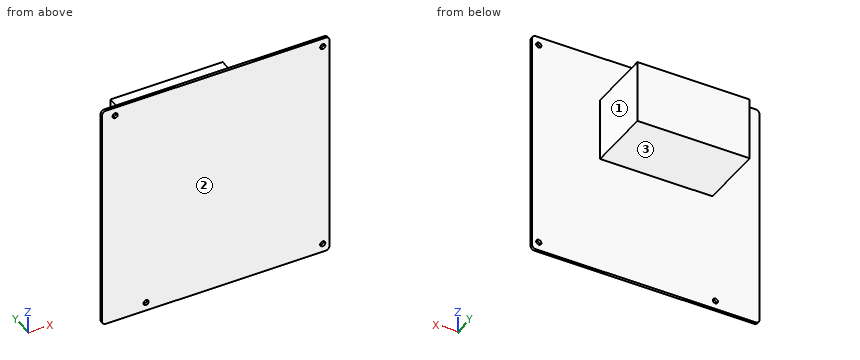
from build123d import *

# Parameters (mm, degrees)
SKETCH1_W                      = 170.18
SKETCH1_H                      = 170.18
BOSS_EXTRUDE1_DEPTH            = 2
SKETCH2_W                      = 84.015738727
SKETCH2_H                      = 47.018762818
BOSS_EXTRUDE2_DEPTH            = 48.8
FILLET1_R                      = 3
F_3_9_3_9_DIAMETER_HOLE1_D     = 3.9
F_3_9_3_9_DIAMETER_HOLE1_DEPTH = 18.75
F_3_9_3_9_DIAMETER_HOLE1_TIP   = 1.171678207


with BuildPart() as part:
    # Sketch1 → Boss-Extrude1 (new body)
    with BuildSketch(Plane(origin=(0, 0, 0), x_dir=(1, 0, 0), z_dir=(0, 1, 0))):
        Rectangle(SKETCH1_W, SKETCH1_H)
    extrude(amount=BOSS_EXTRUDE1_DEPTH)

    # Sketch2 → Boss-Extrude2 (add)
    with BuildSketch(Plane(origin=(0, 2, 0), x_dir=(1, 0, 0), z_dir=(0, 1, 0))):
        with Locations((-7.871346986, -27.578797891)):
            Rectangle(SKETCH2_W, SKETCH2_H)
    extrude(amount=BOSS_EXTRUDE2_DEPTH)

    # Fillet1
    fillet1_edges = [part.edges().sort_by_distance(p)[0] for p in [
        (-85.09, 1, -85.09),
        (85.09, 1, -85.09),
        (85.09, 1, 85.09),
        (-85.09, 1, 85.09),
    ]]
    fillet(fillet1_edges, radius=FILLET1_R)

    # Ø3.9 (3.9) Diameter Hole1
    with Locations(Plane(origin=(0, 2, 0), x_dir=(1, 0, 0), z_dir=(0, 1, 0))):
        with Locations((-75.29, -78.74), (80.01, -78.74), (80.01, 78.74), (-52.07, 78.74)):
            Hole(F_3_9_3_9_DIAMETER_HOLE1_D / 2, depth=F_3_9_3_9_DIAMETER_HOLE1_DEPTH)
            with Locations((0, 0, -(F_3_9_3_9_DIAMETER_HOLE1_DEPTH + F_3_9_3_9_DIAMETER_HOLE1_TIP / 2))):  # 118° drill point
                Cone(0, F_3_9_3_9_DIAMETER_HOLE1_D / 2, F_3_9_3_9_DIAMETER_HOLE1_TIP, mode=Mode.SUBTRACT)


solid = part.part
Geometry: final body of the model. Coordinates: model frame, mm. Face numbers are marked on the shaded views. A direction names the side the tool comes from. Round coordinates to 2 decimals unless told otherwise and drop trailing zeros. Loops run counter-clockwise (first coordinate to the right, second up) from the corner with the lowest first, then second, coordinate; pieces in that order, holes last. Notation, with made-up numbers: (87, 86) -> (140, 86) arc R25 ccw to (140, 120) -> close; hole circle Ø1 at (59, -30.5). An arc over 180 degrees is marked (long way). One line per question, with ' | ' between items. Start each with the question number.
1. Line query: line 1 along X through (y, z) = (1, -78.74); line 2 along Z through (x, y) = (80.01, 1.1); line 3 along Z through (x, y) = (-52.07, 1.4). Output: solid intervals per line, ascending. Write a range as [from, to].
2. Section D-D on x = 57. Output: boundary loops of the cut face in (y, z).
3. Section B-B on z = 37.5. Output: boundary loops of the cut face in (x, y).
4. Set-up query: the marked faces 1, 2 and 3. Return all of +Z, -Z, +X, -X, +Y, -Y with unobstructed straight access to the full face (end or side cutting, diameter ignored); none if empty.
5. Section C-C on y = 24. Output: boundary loops of the cut face in (x, z).
6. Contact query for flat-ended pins moving along their axis: pin 1 (12 mm diameter, centred on x = -17.5, y = 11, fed in from -Z); pin 2 (3 mm diameter, centred on x = -21, z = 56.5, fed in from +Y); pin 3 (3 mm diameter, centred on x = -0.5, y = 10, fed in from +Z). Output: stop coordinate, or through.
7. Section A-A on x = -26. Output: boundary loops of the cut face in (y, z), and give its area (3 significant figures).
Returned:
1) line 1: x = [-85.09, -54.02], [-50.12, 78.06], [81.96, 85.09] | line 2: z = [-85.09, -80.69], [-76.79, 76.79], [80.69, 85.09] | line 3: z = [-85.09, -80.69], [-76.79, 85.09]
2) outline: (0, -85.09) -> (2, -85.09) -> (2, 85.09) -> (0, 85.09) -> close
3) outline: (-85.09, 0) -> (85.09, 0) -> (85.09, 2) -> (34.14, 2) -> (34.14, 50.8) -> (-49.88, 50.8) -> (-49.88, 2) -> (-85.09, 2) -> close
4) face 1: +Z, -Z, +X, +Y | face 2: +Z, -Z, +X, -X, -Y | face 3: -Z, +X, -X, +Y
5) outline: (-49.88, 4.07) -> (34.14, 4.07) -> (34.14, 51.09) -> (-49.88, 51.09) -> close
6) pin 1: stops at z = 4.07 | pin 2: stops at y = 2 | pin 3: stops at z = 51.09
7) outline: (0, -85.09) -> (2, -85.09) -> (2, 4.07) -> (50.8, 4.07) -> (50.8, 51.09) -> (2, 51.09) -> (2, 85.09) -> (0, 85.09) -> close | area: 2,630 mm2
